For this review, use the dimensioned drawing (mm, ordinates from the lowest corner) and the shaded views. A direction names the side the tool comes from. Give positions to 0.01 mm unless a question says otherwise; leave off trailing zeros. Loops run counter-clockwise (first coordinate to the right, second up) from the corner with the lowest first, then second, coordinate; pieces in that order, holes last. Notation, with made-up numbers: (25.25, -14.5) -> (71.25, -14.5) arc R22 ccw to (71.25, 18.5) -> close; hole circle Ø5 at (11, 10.5). An arc over 180 degrees is marked (long way). Use a Markdown table: item, result. Add a question column.
1. Add section C-C (y = 5.75). State the section outline as (x, z) points.
2. Add section A-A (x = 10.42). State the section outline as (y, z) points.
3. Draft analysis for pull direction X (two halves, no side actions). For the marked faces 4, 5 and 6, state which applies: pulls with the +X half, pulls with the -X half, needs draft (parallel to the pull), parting line crosses it, or undercut.
4. Add section D-D (z = 31.5). State the section outline as (x, y) points.
5. To check wall thickness, follow line 1 (Z direction, x = 10.42, y = 6.75); line 2 (Z direction, x = 11.75, y = 8.5); line 3 (Y direction, x = 15.25, z = 10). State the ranges of each line that lie inside material, in increasing order.
6. For pin 1 Ø2 at (y, z) = (2, 23.5) entering from -X; pin 2 Ø3 at (x, z) = (3, 5.5) entering from +Y; pin 3 Ø2 at (x, y) = (7.5, 7.5) entering from -Z; pin 4 Ø1 at (y, z) = (9.5, 20.5) entering from +X, all flat-tipped, find the tip position at first contact; note any pin that passes through.
7. Add section B-B (z = 26). State the section outline as (x, y) points.
8. For the marked faces 1, 2 and 3, list the 3-axis set-ups (+Z, -Z, +X, -X, +Y, -Y) from which the entire face can be reached by the end or side of a thin tool; tool diameter is ignored.
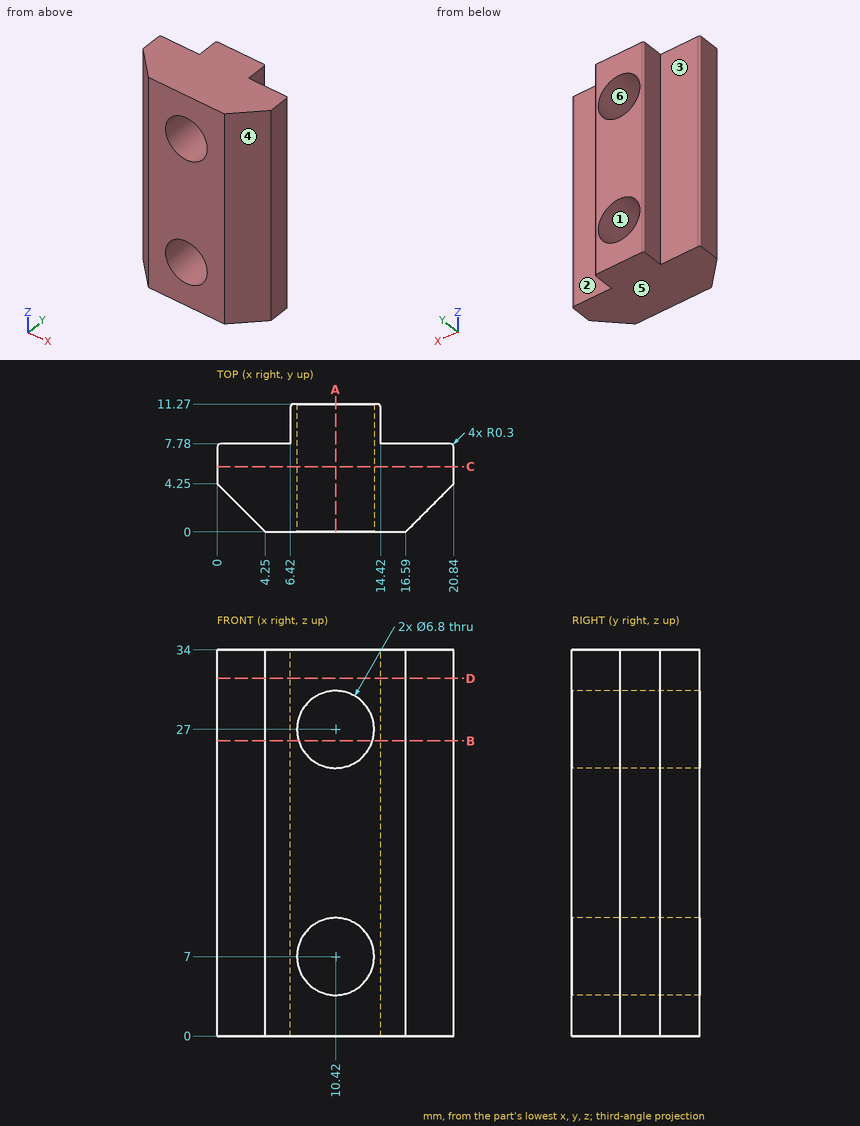
Taken from the geometry:
| question | item | result |
|---|---|---|
| 1 | outline | (0, 0) -> (20.84, 0) -> (20.84, 34) -> (0, 34) -> close; hole circle Ø6.8 at (10.42, 7); hole circle Ø6.8 at (10.42, 27) |
| 2 | outline | (0, 0) -> (11.27, 0) -> (11.27, 3.6) -> (0, 3.6) -> close; (0, 10.4) -> (11.27, 10.4) -> (11.27, 23.6) -> (0, 23.6) -> close; (0, 30.4) -> (11.27, 30.4) -> (11.27, 34) -> (0, 34) -> close |
| 3 | face 4 | pulls with the +X half |
| 3 | face 5 | needs draft |
| 3 | face 6 | undercut |
| 4 | outline | (0, 4.25) -> (4.25, 0) -> (16.59, 0) -> (20.84, 4.25) -> (20.84, 7.48) arc R0.3 ccw to (20.54, 7.78) -> (14.42, 7.78) -> (14.42, 10.97) arc R0.3 ccw to (14.12, 11.27) -> (6.72, 11.27) arc R0.3 ccw to (6.42, 10.97) -> (6.42, 7.78) -> (0.3, 7.78) arc R0.3 ccw to (0, 7.48) -> close |
| 5 | line 1 | z = 0 to 3.6, 10.4 to 23.6, 30.4 to 34 |
| 5 | line 2 | z = 0 to 3.87, 10.13 to 23.87, 30.13 to 34 |
| 5 | line 3 | y = 0 to 7.78 |
| 6 | pin 1 | stops at x = 1.25 |
| 6 | pin 2 | stops at y = 7.78 |
| 6 | pin 3 | stops at z = 0 |
| 6 | pin 4 | stops at x = 14.42 |
| 7 | outline | (0, 4.25) -> (4.25, 0) -> (7.17, 0) -> (7.17, 11.27) -> (6.72, 11.27) arc R0.3 ccw to (6.42, 10.97) -> (6.42, 7.78) -> (0.3, 7.78) arc R0.3 ccw to (0, 7.48) -> close; (13.67, 0) -> (16.59, 0) -> (20.84, 4.25) -> (20.84, 7.48) arc R0.3 ccw to (20.54, 7.78) -> (14.42, 7.78) -> (14.42, 10.97) arc R0.3 ccw to (14.12, 11.27) -> (13.67, 11.27) -> close |
| 8 | face 1 | +Y, -Y |
| 8 | face 2 | +Z, -Z, +X, +Y |
| 8 | face 3 | +Z, -Z, -X, +Y |
